Can you work these out from the model? Positions are in its coordinate system, mm. A direction names the side the tool comes from. Give positions to 0.01 mm unless a question says otherwise; leave off trailing zeros. Write each loop counter-clockwise with the first axis right and the second up, starting at its lowest first coordinate (ties: lowest second). Pieces come first, ordered by that corner, then holes. Notation, with made-up numbers: (4.25, 88) - (59.25, 88) arc R24 ccw to (59.25, 120) - close; hole circle Ø8 at (38, 53.25). An arc over 180 degrees is marked (long way). Use a Markdown table: item, result. Add a question column.
```python
from build123d import *

# Parameters (mm, degrees)
EXTRUDE_1_DEPTH      = 15
SKETCH_2_R           = 35
EXTRUDE_2_DEPTH      = 10
SKETCH_3_R           = 65
SKETCH_3_R_2         = 50
EXTRUDE_3_DEPTH      = 10
SKETCH_4_R           = 25
CUT_EXTRUDE_1_DEPTH  = 20
CUT_EXTRUDE_2_REACH  = 124.78
SKETCH_5_R           = 6.75
EXTRUDE_4_REACH      = 193.703
EXTRUDE_4_END_RADIUS = 35
SKETCH_9_R           = 10
SKETCH_11_R          = 3
SKETCH_10_R          = 6
SKETCH_12_R          = 3
CUT_EXTRUDE_4_DEPTH  = 33
SKETCH_13_R          = 3
CUT_EXTRUDE_5_DEPTH  = 13
EXTRUDE_START        = 6
EXTRUDE_5_DEPTH      = 6
EXTRUDE_6_DEPTH      = 13
M10X1_52_D           = 8.5
M10X1_52_DEPTH       = 18
M10X1_52_CSINK_D     = 10.05
M10X1_52_CSINK_ANGLE = 90
M10X1_52_TIP         = 2.553657631


with BuildPart() as part:
    # Эскиз1 → Бобышка-Вытянуть1 (new body)
    with BuildSketch(Plane(origin=(0, 0, 0), x_dir=(1, 0, 0), z_dir=(0, 1, 0))):
        with BuildLine():
            Line((-65, -85), (65, -85))
            ThreePointArc((65, -85), (79.142135624, -79.142135624), (85, -65))
            Line((85, -65), (85, 65))
            ThreePointArc((85, 65), (79.142135624, 79.142135624), (65, 85))
            Line((65, 85), (-65, 85))
            ThreePointArc((-65, 85), (-79.142135624, 79.142135624), (-85, 65))
            Line((-85, 65), (-85, -65))
            ThreePointArc((-85, -65), (-79.142135624, -79.142135624), (-65, -85))
        make_face()
    extrude(amount=EXTRUDE_1_DEPTH)

    # Эскиз2 → Бобышка-Вытянуть2 (add)
    with BuildSketch(Plane(origin=(0, 15, 0), x_dir=(1, 0, 0), z_dir=(0, 1, 0))):
        with Locations(Location((0, 0, 0), (0, 0, 270))):
            Circle(SKETCH_2_R)
    extrude(amount=EXTRUDE_2_DEPTH)

    # Эскиз3 → Бобышка-Вытянуть3 (add)
    with BuildSketch(Plane.XZ):
        with Locations(Location((0, 0, 0), (0, 0, 90))):
            Circle(SKETCH_3_R)
        with Locations(Location((0, 0, 0), (0, 0, 270))):
            Circle(SKETCH_3_R_2, mode=Mode.SUBTRACT)
    extrude(amount=EXTRUDE_3_DEPTH)

    # Эскиз4 → Вырез-Вытянуть1 (cut)
    with BuildSketch(Plane(origin=(0, 25, 0), x_dir=(1, 0, 0), z_dir=(0, 1, 0))):
        with Locations(Location((0, 0, 0), (0, 0, 270))):
            Circle(SKETCH_4_R)
    extrude(amount=-CUT_EXTRUDE_1_DEPTH, mode=Mode.SUBTRACT)

    # Эскиз5 → Вырез-Вытянуть2 (cut, up to next)
    with BuildSketch(Plane(origin=(0, 15, 0), x_dir=(1, 0, 0), z_dir=(0, 1, 0)), mode=Mode.PRIVATE) as cut_extrude_2_sk1:
        with Locations(Location((-62.5, 62.5, 0), (0, 0, 270))):
            Circle(SKETCH_5_R)
    cut_extrude_2_tool1 = extrude(cut_extrude_2_sk1.sketch, amount=-CUT_EXTRUDE_2_REACH, mode=Mode.PRIVATE) & part.part
    # Эскиз5 → Вырез-Вытянуть2 (cut, up to next)
    with BuildSketch(Plane(origin=(0, 15, 0), x_dir=(1, 0, 0), z_dir=(0, 1, 0)), mode=Mode.PRIVATE) as cut_extrude_2_sk2:
        with Locations(Location((62.5, 62.5, 0), (0, 0, 270))):
            Circle(SKETCH_5_R)
    cut_extrude_2_tool2 = extrude(cut_extrude_2_sk2.sketch, amount=-CUT_EXTRUDE_2_REACH, mode=Mode.PRIVATE) & part.part
    # Эскиз5 → Вырез-Вытянуть2 (cut, up to next)
    with BuildSketch(Plane(origin=(0, 15, 0), x_dir=(1, 0, 0), z_dir=(0, 1, 0)), mode=Mode.PRIVATE) as cut_extrude_2_sk3:
        with Locations(Location((62.5, -62.5, 0), (0, 0, 270))):
            Circle(SKETCH_5_R)
    cut_extrude_2_tool3 = extrude(cut_extrude_2_sk3.sketch, amount=-CUT_EXTRUDE_2_REACH, mode=Mode.PRIVATE) & part.part
    # Эскиз5 → Вырез-Вытянуть2 (cut, up to next)
    with BuildSketch(Plane(origin=(0, 15, 0), x_dir=(1, 0, 0), z_dir=(0, 1, 0)), mode=Mode.PRIVATE) as cut_extrude_2_sk4:
        with Locations(Location((-62.5, -62.5, 0), (0, 0, 270))):
            Circle(SKETCH_5_R)
    cut_extrude_2_tool4 = extrude(cut_extrude_2_sk4.sketch, amount=-CUT_EXTRUDE_2_REACH, mode=Mode.PRIVATE) & part.part
    add(cut_extrude_2_tool1.solids().sort_by_distance((-62.5, 15, -62.5))[0], mode=Mode.SUBTRACT)
    add(cut_extrude_2_tool2.solids().sort_by_distance((62.5, 15, -62.5))[0], mode=Mode.SUBTRACT)
    add(cut_extrude_2_tool3.solids().sort_by_distance((62.5, 15, 62.5))[0], mode=Mode.SUBTRACT)
    add(cut_extrude_2_tool4.solids().sort_by_distance((-62.5, 15, 62.5))[0], mode=Mode.SUBTRACT)

    # Бобышка-Вытянуть4: up to this cylinder (the profile starts outside it)
    extrude_4_end = Plane(origin=(0, 10, 0), z_dir=(0, -1, 0)) * Cylinder(EXTRUDE_4_END_RADIUS, 458.406, mode=Mode.PRIVATE)
    # Эскиз9 → Бобышка-Вытянуть4 (add, up to the surface)
    with BuildSketch(Plane(origin=(0, 0, -85), x_dir=(-1, 0, 0), z_dir=(0, 0, -1)), mode=Mode.PRIVATE) as extrude_4_sk1:
        with Locations((0, 10)):
            Circle(SKETCH_9_R)
    extrude_4_tool1 = extrude(extrude_4_sk1.sketch, amount=-EXTRUDE_4_REACH, mode=Mode.PRIVATE) - extrude_4_end
    add(extrude_4_tool1.solids().sort_by_distance((0, 10, -85))[0])

    # Эскиз11 → Вырез-По сечениям1 section 0
    with BuildSketch(Plane(origin=(0, 0, -73), x_dir=(-1, 0, 0), z_dir=(0, 0, -1))):
        with Locations((0, 10)):
            Circle(SKETCH_11_R)
    # Эскиз10 → Вырез-По сечениям1 section 1
    with BuildSketch(Plane(origin=(0, 0, -85), x_dir=(-1, 0, 0), z_dir=(0, 0, -1))):
        with Locations((0, 10)):
            Circle(SKETCH_10_R)
    loft(mode=Mode.SUBTRACT)

    # Эскиз12 → Вырез-Вытянуть4 (cut)
    with BuildSketch(Plane(origin=(0, 0, -73), x_dir=(-1, 0, 0), z_dir=(0, 0, -1))):
        with Locations((0, 10)):
            Circle(SKETCH_12_R)
    extrude(amount=-CUT_EXTRUDE_4_DEPTH, mode=Mode.SUBTRACT)

    # Эскиз13 → Вырез-Вытянуть5 (cut)
    with BuildSketch(Plane.XZ):
        with Locations(Location((0, -43, 0), (0, 0, 270))):
            Circle(SKETCH_13_R)
    extrude(amount=-CUT_EXTRUDE_5_DEPTH, mode=Mode.SUBTRACT)

    # Эскиз14 → Бобышка-Вытянуть5 (add)
    with BuildSketch(Plane(origin=(0, 0, -40), x_dir=(-1, 0, 0), z_dir=(0, 0, -1)).offset(EXTRUDE_START)):
        with BuildLine():
            Line((3, 10), (4.5, 10))
            ThreePointArc((4.5, 10), (0, 14.5), (-4.5, 10))
            Line((-4.5, 10), (-3, 10))
            ThreePointArc((-3, 10), (0, 13), (3, 10))
        make_face()
    extrude(amount=-EXTRUDE_5_DEPTH)

    # Эскиз15 → Бобышка-Вытянуть6 (add)
    with BuildSketch(Plane.XZ):
        with BuildLine():
            Line((-3, -43), (-4.5, -43))
            ThreePointArc((-4.5, -43), (0, -38.5), (4.5, -43))
            Line((4.5, -43), (3, -43))
            ThreePointArc((3, -43), (0, -40), (-3, -43))
        make_face()
    extrude(amount=-EXTRUDE_6_DEPTH)

    # Отверстие обработанное метчиком M10x1.52
    with Locations(Plane(origin=(-40, 15, -40), x_dir=(0, 0, 1), z_dir=(0, 1, 0))):
        with Locations((0, 0), (0, 80), (80, 80), (80, 0)):
            CounterSinkHole(M10X1_52_D / 2, M10X1_52_CSINK_D / 2, depth=M10X1_52_DEPTH, counter_sink_angle=M10X1_52_CSINK_ANGLE)
            with Locations((0, 0, -(M10X1_52_DEPTH + M10X1_52_TIP / 2))):  # 118° drill point
                Cone(0, M10X1_52_D / 2, M10X1_52_TIP, mode=Mode.SUBTRACT)


solid = part.part
```
Q1. If I drill on probe 1 along Z at (x, y) = (40, 8); probe 2 along X at (y, z) = (6, -62), over which ranges is the centre line in solid material (lowest first)? Write a range as [from, to].
Q2. Suppose I cut it at B-B (x = -62.5). Please give me the cut outline in (y, z).
Q3. If we mould it in two halves opening along X, with no side actions, what happens to faces 1 (the cylindrical face through (-78.986, 7.395, -79.297)), 2 (the flat face through (37, 0, 55)), 3 (the cylindrical face through (40.187, 5.492, 44.246))? For each: released by +X, released by -X, zero draft, split by the parting line, or undercut.
Q4. Suppose I cut it at C-C (z = 0). Please give me the cut outline in (x, y), and give its area (3 significant figures).
Q5. I'm going to push flat-ended pins straight in: P1, Ø17.5, axis at x = 62.5, z = 62.5, coming from the -Y side; P2, Ø8, axis at x = -62.5, z = -62.5, coming from the -Y side; P3, Ø6, axis at y = 20.5, z = 4, coming from the +X side; P4, Ø10, axis at x = -64, z = 43, coming from the +Y side. Where does each tip first touch, or does it pass through?
Q6. Suppose I cut it at D-D (x = 13). Please give me the cut outline in (y, z), and give its area (3 significant figures).
Q7. On a 3-axis mill with a long thin cutter (end or side, diameter ignored), from which of +Z, -Z, +X, -X, +Y, -Y can I reach the whole of each face in a straight line? I mean faces 4 (the cylindrical face through (10.513, 19.93, 33.384)), 5 (the flat face through (-1, 7, 85)). Say none if no direction works.
Q8. Suppose I cut it at A-A (z = -62.5). Please give me the cut outline in (x, y).
Derived:
| question | item | result |
|---|---|---|
| 1 | probe 1 | [-85, -44.25], [-35.75, 35.75], [44.25, 85] |
| 1 | probe 2 | [-85, -69.23], [-55.77, 55.77], [69.23, 85] |
| 2 | outline | (-10, -17.85) - (0, -17.85) - (0, -55.75) - (15, -55.75) - (15, 55.75) - (0, 55.75) - (0, 17.85) - (-10, 17.85) - close; (0, -85) - (15, -85) - (15, -69.25) - (0, -69.25) - close; (0, 69.25) - (15, 69.25) - (15, 85) - (0, 85) - close |
| 3 | face 1 | released by -X |
| 3 | face 2 | zero draft |
| 3 | face 3 | undercut |
| 4 | outline | (-85, 0) - (-65, 0) - (-65, -10) - (-50, -10) - (-50, 0) - (50, 0) - (50, -10) - (65, -10) - (65, 0) - (85, 0) - (85, 15) - (35, 15) - (35, 25) - (25, 25) - (25, 5) - (-25, 5) - (-25, 25) - (-35, 25) - (-35, 15) - (-85, 15) - close |
| 4 | area | 2,550 mm² |
| 5 | P1 | y = 0 |
| 5 | P2 | through |
| 5 | P3 | x = 34.99 |
| 5 | P4 | y = 15 |
| 6 | outline | (-10, -63.69) - (0, -63.69) - (0, -85) - (15, -85) - (15, -32.5) - (25, -32.5) - (25, -21.35) - (5, -21.35) - (5, 21.35) - (25, 21.35) - (25, 32.5) - (15, 32.5) - (15, 85) - (0, 85) - (0, 63.69) - (-10, 63.69) - (-10, 48.28) - (0, 48.28) - (0, -48.28) - (-10, -48.28) - close |
| 6 | area | 2,650 mm² |
| 7 | face 4 | +Y |
| 7 | face 5 | +Z, +X, -X, +Y, -Y |
| 8 | outline | (-85, 0) - (-69.25, 0) - (-69.25, 15) - (-85, 15) - close; (-55.75, 0) - (-17.85, 0) - (-17.85, -10) - (17.85, -10) - (17.85, 0) - (55.75, 0) - (55.75, 15) - (8.66, 15) arc R10 ccw to (-8.66, 15) - (-55.75, 15) - close; (69.25, 0) - (85, 0) - (85, 15) - (69.25, 15) - close; hole circle Ø6 at (0, 10) |
